```python
from build123d import *

# Parameters (mm, degrees)
ESQUISSE1_R             = 5.4
BOSS_EXTRU_1_DEPTH      = 3
ESQUISSE2_R             = 3.85
BOSS_EXTRU_2_DEPTH      = 5.5
ESQUISSE3_R             = 4
BOSS_EXTRU_3_DEPTH      = 6.4
ESQUISSE4_W             = 3
ESQUISSE4_H             = 0.5
ESQUISSE4_W_2           = 0.5
ESQUISSE4_H_2           = 3
BOSS_EXTRU_4_DEPTH      = 6.5
ESQUISSE5_R             = 3
ENL_V_MAT_EXTRU_1_DEPTH = 10
ESQUISSE6_R             = 1
BOSS_EXTRU_5_DEPTH      = 8


with BuildPart() as part:
    # Esquisse1 → Boss.-Extru.1 (new body)
    with BuildSketch(Plane(origin=(0, 0, 0), x_dir=(1, 0, 0), z_dir=(0, 1, 0))):
        Circle(ESQUISSE1_R)
    extrude(amount=BOSS_EXTRU_1_DEPTH)

    # Esquisse2 → Boss.-Extru.2 (add)
    with BuildSketch(Plane(origin=(0, 3, 0), x_dir=(1, 0, 0), z_dir=(0, 1, 0))):
        Circle(ESQUISSE2_R)
    extrude(amount=BOSS_EXTRU_2_DEPTH)

    # Esquisse3 → Boss.-Extru.3 (add)
    with BuildSketch(Plane.XZ):
        Circle(ESQUISSE3_R)
    extrude(amount=BOSS_EXTRU_3_DEPTH)

    # Esquisse4 → Boss.-Extru.4 (add)
    with BuildSketch(Plane.XZ.offset(6.4)):
        with Locations((0.005129852, -3.453606957)):
            Rectangle(ESQUISSE4_W, ESQUISSE4_H)
        with Locations((0.005129852, 3.453606957)):
            Rectangle(ESQUISSE4_W, ESQUISSE4_H)
        with Locations((3.458099244, 0)):
            Rectangle(ESQUISSE4_W_2, ESQUISSE4_H_2)
    extrude(amount=BOSS_EXTRU_4_DEPTH)

    # Esquisse5 → Enlèv. mat.-Extru.1 (cut)
    with BuildSketch(Plane(origin=(0, 8.5, 0), x_dir=(1, 0, 0), z_dir=(0, 1, 0))):
        Circle(ESQUISSE5_R)
    extrude(amount=-ENL_V_MAT_EXTRU_1_DEPTH, mode=Mode.SUBTRACT)

    # Esquisse6 → Boss.-Extru.5 (add)
    with BuildSketch(Plane(origin=(0, -1.5, 0), x_dir=(1, 0, 0), z_dir=(0, 1, 0))):
        Circle(ESQUISSE6_R)
    extrude(amount=BOSS_EXTRU_5_DEPTH)


solid = part.part
```
Work out the finished part from the listing and answer in its coordinate system (mm). A direction names the side the tool comes from. Round coordinates to 2 decimals unless told otherwise and drop trailing zeros. Loops run counter-clockwise (first coordinate to the right, second up) from the corner with the lowest first, then second, coordinate; pieces in that order, holes last.
(1) The part is cut by section B-B, the plane z = 0. Give the vertices of the cut face in (x, y), and give its area (3 significant figures).
Computed values:
outline: (-5.4, 0) - (-4, 0) - (-4, -6.4) - (3.21, -6.4) - (3.21, -12.9) - (3.71, -12.9) - (3.71, -6.4) - (4, -6.4) - (4, 0) - (5.4, 0) - (5.4, 3) - (3.85, 3) - (3.85, 8.5) - (3, 8.5) - (3, -1.5) - (1, -1.5) - (1, 6.5) - (-1, 6.5) - (-1, -1.5) - (-3, -1.5) - (-3, 8.5) - (-3.85, 8.5) - (-3.85, 3) - (-5.4, 3) - close
area: 85.2 mm2
(2) The part is cut by section A-A, the plane y = -10.5. Give the vertices of the cut face in (x, z).
Computed values:
outline: (-1.49, -3.7) - (1.51, -3.7) - (1.51, -3.2) - (-1.49, -3.2) - close; (-1.49, 3.2) - (1.51, 3.2) - (1.51, 3.7) - (-1.49, 3.7) - close; (3.21, -1.5) - (3.71, -1.5) - (3.71, 1.5) - (3.21, 1.5) - close
(3) The mould has two halves that part along X. Classify faces 1 (the cylindrical face through (-3, 4, 0)), 2 (the flat face through (0, -6.4, 0)), 3 (the cylindrical face through (-1.17, 1.48, 5.27)): pulls with the +X half, pulls with the -X half, needs draft (parallel to the pull), parting line crosses it, or undercut.
Computed values:
face 1: undercut
face 2: needs draft
face 3: parting line crosses it
(4) Each of these flat-tipped pins is pushed along its axis until it touches: P1, Ø0.9, axis at x = 0, y = -9.5, coming from the +Z side; P2, Ø0.6, axis at x = 0.5, z = -0.5, coming from the +Y side; P3, Ø0.9, axis at x = 0.5, y = -8, coming from the -Z side. Where does it stop, or does it pass through?
Computed values:
P1: stops at z = 3.7
P2: stops at y = 6.5
P3: stops at z = -3.7
(5) Find the intervals of material crossed by L1, parallel to X at y = 4, z = 0; L2, parallel to Z at x = 0, y = 1.5, in increasing order.
Computed values:
L1: x = -3.85 to -3, -1 to 1, 3 to 3.85
L2: z = -5.4 to -3, -1 to 1, 3 to 5.4
(6) For faces 4 (the cylindrical face through (-0.867, -3.155, -3.905)), 5 (the flat face through (0, -10, -3.704)), 6 (the flat face through (0, -10, 3.704)), 7 (the cylindrical face through (0, 2, 1)), 8 (the flat face through (0, -10, -3.204)), determine the directions among +Z, -Z, +X, -X, +Y, -Y from which every point of the face is accessible in a straight line to the end or side of a thin tool.
Computed values:
face 4: -Y
face 5: -Z, +X, -X, -Y
face 6: +Z, +X, -X, -Y
face 7: +Y
face 8: +X, -X, -Y
(7) The part is cut by section C-C, the plane x = 0. Give the vertices of the cut face in (y, z), and give its area (4 significant figures).
Computed values:
outline: (-12.9, -3.7) - (-6.4, -3.7) - (-6.4, -4) - (0, -4) - (0, -5.4) - (3, -5.4) - (3, -3.85) - (8.5, -3.85) - (8.5, -3) - (-1.5, -3) - (-1.5, -1) - (6.5, -1) - (6.5, 1) - (-1.5, 1) - (-1.5, 3) - (8.5, 3) - (8.5, 3.85) - (3, 3.85) - (3, 5.4) - (0, 5.4) - (0, 4) - (-6.4, 4) - (-6.4, 3.7) - (-12.9, 3.7) - (-12.9, 3.2) - (-6.4, 3.2) - (-6.4, -3.2) - (-12.9, -3.2) - close
area: 88.45 mm2
(8) The part is cut by section D-D, the plane y = -1. Give the vertices of the cut face in (x, z), and give its area (3 significant figures).
Computed values:
outline: circle Ø8 at (0, 0); circle Ø2 at (0, 0); hole circle Ø6 at (0, 0)
area: 25.1 mm2
